from build123d import *

# Parameters (mm, degrees)
F4_DEPTH       = 10.29
F1_W           = 7.18
F1_H           = 5.9
F5_DEPTH       = 6.02
F1_W_2         = 14.75
F1_H_2         = 15.15
F1_W_3         = 10.47
F1_H_3         = 10.1
F6_DEPTH       = 5.94
F1_W_4         = 15.6
F1_H_4         = 15.6
F7_DEPTH       = 0.8
F8_DEPTH       = 7.801
F8_DEPTH_BACK  = 7.801
F9_DEPTH       = 7.801
F9_DEPTH_BACK  = 7.801
F0_W           = 13.95
F0_H           = 13.9
F0_R           = 0.4953
F0_R_2         = 0.7493
F0_R_3         = 1.9939
F10_DEPTH      = 4.71
F11_DEPTH      = 7.54
F12_DEPTH      = 8.1
F13_DEPTH      = 5.23
F14_DEPTH      = 7.801
F14_DEPTH_BACK = 7.801


with BuildPart() as f4:
    # F1 (on Top) → F4 (new body, through all)
    with BuildSketch(Plane.XY):
        Polygon((0.55, 2), (-0.55, 2), (-0.55, 0.645), (-1.905, 0.645), (-1.905, -0.645), (-0.55, -0.645), (-0.55, -2), (0.55, -2), (0.55, -0.645), (1.905, -0.645), (1.905, 0.645), (0.55, 0.645), align=None)
    extrude(amount=F4_DEPTH)

    # F1 (on Top) → F5 (join, through all)
    with BuildSketch(Plane.XY):
        Rectangle(F1_W, F1_H)
        Polygon((-0.55, 0.645), (-0.55, 2), (0.55, 2), (0.55, 0.645), (1.905, 0.645), (1.905, -0.645), (0.55, -0.645), (0.55, -2), (-0.55, -2), (-0.55, -0.645), (-1.905, -0.645), (-1.905, 0.645), align=None, mode=Mode.SUBTRACT)
    extrude(amount=F5_DEPTH)

    # F1 (on Top) → F6 (join, through all)
    with BuildSketch(Plane.XY):
        Rectangle(F1_W_2, F1_H_2)
        with Locations((0, 1.1)):
            Rectangle(F1_W_3, F1_H_3, mode=Mode.SUBTRACT)
        with Locations((0, 1.1)):
            Rectangle(F1_W_3, F1_H_3)
        Rectangle(F1_W, F1_H, mode=Mode.SUBTRACT)
    extrude(amount=F6_DEPTH)

    # F1 (on Top) → F7 (join, through all)
    with BuildSketch(Plane.XY):
        Rectangle(F1_W_4, F1_H_4)
        Rectangle(F1_W_2, F1_H_2, mode=Mode.SUBTRACT)
    extrude(amount=F7_DEPTH)

    # F2 (on Right) → F8 (cut, two sides)
    with BuildSketch(Plane.YZ) as f8_sk:
        Polygon((-7.8, 5.94), (-7.8, 0.8), (-7.575, 0.8), (-3.95, 5.94), align=None)
        Polygon((6.15, 5.94), (7.575, 0.8), (7.8, 0.8), (7.8, 5.94), align=None)
    extrude(amount=-F8_DEPTH, mode=Mode.SUBTRACT)
    extrude(f8_sk.sketch, amount=F8_DEPTH_BACK, mode=Mode.SUBTRACT)

    # F3 (on Front) → F9 (cut, two sides)
    with BuildSketch(Plane.XZ) as f9_sk:
        Polygon((-7.8, 5.94), (-7.8, 0.8), (-7.375, 0.8), (-5.235, 5.94), align=None)
        Polygon((5.235, 5.94), (7.375, 0.8), (7.8, 0.8), (7.8, 5.94), align=None)
    extrude(amount=-F9_DEPTH, mode=Mode.SUBTRACT)
    extrude(f9_sk.sketch, amount=F9_DEPTH_BACK, mode=Mode.SUBTRACT)

    # F0 (on Top) → F10 (join, through all)
    with BuildSketch(Plane.XY):
        Rectangle(F0_W, F0_H)
        with Locations((-3.81, -5.08)):
            Circle(F0_R, mode=Mode.SUBTRACT)
        with Locations((3.81, -5.08)):
            Circle(F0_R, mode=Mode.SUBTRACT)
        with Locations((-3.81, 2.54)):
            Circle(F0_R_2, mode=Mode.SUBTRACT)
        Circle(F0_R_3, mode=Mode.SUBTRACT)
        with Locations((2.54, 5.08)):
            Circle(F0_R_2, mode=Mode.SUBTRACT)
    extrude(amount=-F10_DEPTH)

    # F0 (on Top) → F11 (join, through all)
    with BuildSketch(Plane.XY):
        Circle(F0_R_3)
    extrude(amount=-F11_DEPTH)

    # F0 (on Top) → F12 (join, through all)
    with BuildSketch(Plane.XY):
        with Locations((-3.81, 2.54)):
            Circle(F0_R_2)
        with Locations((2.54, 5.08)):
            Circle(F0_R_2)
    extrude(amount=-F12_DEPTH)

    # F0 (on Top) → F13 (join, through all)
    with BuildSketch(Plane.XY):
        with Locations((3.81, -5.08)):
            Circle(F0_R)
        with Locations((-3.81, -5.08)):
            Circle(F0_R)
    extrude(amount=-F13_DEPTH)

    # F3 (on Front) → F14 (cut, two sides)
    with BuildSketch(Plane.XZ) as f14_sk:
        Polygon((-6.975, 0), (-7.8, 0), (-7.8, -4.71), (-6.23, -4.71), align=None)
        Polygon((7.8, 0), (6.975, 0), (6.23, -4.71), (7.8, -4.71), align=None)
    extrude(amount=-F14_DEPTH, mode=Mode.SUBTRACT)
    extrude(f14_sk.sketch, amount=F14_DEPTH_BACK, mode=Mode.SUBTRACT)


solid = f4.part
Can you work these out from the model? Positions are in its coordinate system, mm. A direction names the side the tool comes from. Give positions to 0.01 mm unless a question says otherwise; leave off trailing zeros. Write each loop counter-clockwise with the first axis right and the second up, starting at its lowest first coordinate (ties: lowest second). Pieces come first, ordered by that corner, then holes. Notation, with made-up numbers: (15, 28.25) -> (46, 28.25) arc R19 ccw to (46, 63.25) -> close; hole circle Ø11 at (69.25, 60.25). An arc over 180 degrees is marked (long way). Answer as a JSON object with one key per item and string values. Group by question number.
Item 1: Suppose I cut it at B-B (z = 7.25). Please give me the cut outline in (x, y) (3 decimals).
Item 2: We'd pull the mould along X, two halves only. Please class faces 5 (the face through (2.38, 4.35, -6.38)), 6 (the face through (0, 6.95, -2)), 7 (the face through (3.44, -4.75, -4.97)): +X half, -X half, draft (parallel to the pull), parting line (faces both ways), or undercut.
Item 3: Suppose I cut it at D-D (y = 2.54). Please give me the cut outline in (x, z) (3 decimals).
Item 4: Suppose I cut it at A-A (y = 0). Please give me the cut outline in (x, z) (3 decimals), plus the area to 3 significant figures.
Item 5: I'm going to push flat-ended pins straight in: P1, Ø4.5, axis at x = 0, y = -0.5, coming from the -Z side; P2, Ø1.1, axis at x = 4, y = -5, coming from the -Z side; P3, Ø1, axis at x = -2.5, z = 3, coming from the -Y side. Where does each tip first touch, or does it pass through?
Item 6: Please list where these lines run through material, in increasing order: line 1 (Z direction, x = 4, y = 0.5); line 2 (Z direction, x = 3.5, y = -2.5); line 3 (Y direction, x = -6.5, z = -2.25). Write a range as [from, to].
Item 7: For faces 1 (the face through (1, 0.645, 8)), 2 (the face through (-4.56, 2.57, -6.38)), 3 (the face through (0, -2, 8)), 4 (the face through (0, 2, 8)), which set-ups out of +Z, -Z, +X, -X, +Y, -Y let a thin tool reach every point of the face, with its end or its side?
Item 8: Suppose I cut it at C-C (x = 0). Please give me the cut outline in (y, z) (3 decimals), plus the area to 3 significant figures.
Findings:
{
 "1": {"outline": "(-1.905, -0.645) -> (-0.55, -0.645) -> (-0.55, -2) -> (0.55, -2) -> (0.55, -0.645) -> (1.905, -0.645) -> (1.905, 0.645) -> (0.55, 0.645) -> (0.55, 2) -> (-0.55, 2) -> (-0.55, 0.645) -> (-1.905, 0.645) -> close"},
 "2": {"face 5": "parting line", "face 6": "draft", "face 7": "undercut"},
 "3": {"outline": "(-7.8, 0) -> (-6.975, 0) -> (-6.23, -4.71) -> (-4.559, -4.71) -> (-4.559, -8.1) -> (-3.061, -8.1) -> (-3.061, -4.71) -> (6.23, -4.71) -> (6.975, 0) -> (7.8, 0) -> (7.8, 0.8) -> (7.375, 0.8) -> (5.235, 5.94) -> (3.59, 5.94) -> (3.59, 6.02) -> (-3.59, 6.02) -> (-3.59, 5.94) -> (-5.235, 5.94) -> (-7.375, 0.8) -> (-7.8, 0.8) -> close"},
 "4": {"outline": "(-7.8, 0) -> (-6.975, 0) -> (-6.23, -4.71) -> (-1.994, -4.71) -> (-1.994, -7.54) -> (1.994, -7.54) -> (1.994, -4.71) -> (6.23, -4.71) -> (6.975, 0) -> (7.8, 0) -> (7.8, 0.8) -> (7.375, 0.8) -> (5.235, 5.94) -> (3.59, 5.94) -> (3.59, 6.02) -> (1.905, 6.02) -> (1.905, 10.29) -> (-1.905, 10.29) -> (-1.905, 6.02) -> (-3.59, 6.02) -> (-3.59, 5.94) -> (-5.235, 5.94) -> (-7.375, 0.8) -> (-7.8, 0.8) -> close", "area": "168 mm²"},
 "5": {"P1": "stops at z = -7.54", "P2": "stops at z = -5.23", "P3": "stops at y = -6.38"},
 "6": {"line 1": "z = [-4.71, 5.94]", "line 2": "z = [-4.71, 6.02]", "line 3": "y = [-6.95, 6.95]"},
 "7": {"face 1": "+Z, +X, +Y", "face 2": "-Z", "face 3": "+Z, +X, -X, -Y", "face 4": "+Z, +X, -X, +Y"},
 "8": {"outline": "(-7.8, 0) -> (-6.95, 0) -> (-6.95, -4.71) -> (-1.994, -4.71) -> (-1.994, -7.54) -> (1.994, -7.54) -> (1.994, -4.71) -> (6.95, -4.71) -> (6.95, 0) -> (7.8, 0) -> (7.8, 0.8) -> (7.575, 0.8) -> (6.15, 5.94) -> (2.95, 5.94) -> (2.95, 6.02) -> (2, 6.02) -> (2, 10.29) -> (-2, 10.29) -> (-2, 6.02) -> (-2.95, 6.02) -> (-2.95, 5.94) -> (-3.95, 5.94) -> (-7.575, 0.8) -> (-7.8, 0.8) -> close", "area": "172 mm²"}
}
